For this review, take the finished solid that the model builds, in its own axes (mm). A direction names the side the tool comes from. Coordinates: 2 decimals unless noted, no trailing zeros. Order: outer loops, then holes, each group sorted by start corner. A loop starts at its lowest first (then second) coordinate and runs counter-clockwise, first axis right, second up. Notation, with made-up numbers: M -19,80.5 L -2,80.5 A23 cw -2,95.5 Z; hole C 2,74 d9. An arc over 180 degrees is marked long. Use CSV: the item, a comma, the result in double quotes.
```python
from build123d import *

# Parameters (mm, degrees)
F0_W      = 37.8
F0_H      = 23.2
F1_DEPTH  = 3
F3_DEPTH  = 4.5
F4_W      = 30
F4_H      = 13.9
F5_DEPTH  = 25.4
F4_W_2    = 34.5051246695
F4_H_2    = 1.524
F6_DEPTH  = 0.5
F7_R      = 0.25
F8_R      = 0.2
F9_R      = 0.2
F11_DEPTH = 5.5
F12_R     = 2.19964
F13_R     = 2.19964
F15_R     = 1.2
F14_R     = 1.2
F16_DEPTH = 25.4


with BuildPart() as f1:
    # F0 (on Top) → F1 (new body)
    with BuildSketch(Plane.XY):
        with Locations((18.9, 11.6)):
            Rectangle(F0_W, F0_H)
    extrude(amount=F1_DEPTH)

    # F2 (on face) → F3 (join)
    with BuildSketch(Plane.XY.offset(3)):
        Polygon((1.7535259355, 24.5575234294), (3.1678657052, 23.2), (3.544374615, 23.2), (2.1300348453, 24.5575234294), align=None)
        Polygon((3.544374615, 23.2), (3.1678657052, 23.2), (4.5401435345, 21.8828488141), (4.8160737062, 21.97938714), align=None)
        Polygon((2.5074673859, 0), (1.9109652349, 0), (1.0702608852, -0.7231329801), (1.3239181902, -1.0180314366), align=None)
        Polygon((4.5401435345, 1.7484091301), (4.5401435345, 2.2614912596), (1.9109652349, 0), (2.5074673859, 0), align=None)
        Polygon((33.6620093499, 2.2614912596), (35.6072341062, 0), (35.9434980693, 0), (33.998273313, 2.2614912596), align=None)
        Polygon((35.9434980693, 0), (35.6072341062, 0), (36.2292379141, -0.7231329801), (36.5655018772, -0.7231329801), align=None)
        Polygon((36.2128205597, 24.5575234294), (34.9098310654, 23.2), (35.2625123829, 23.2), (36.5655018772, 24.5575234294), align=None)
        Polygon((35.2625123829, 23.2), (34.9098310654, 23.2), (33.6403721345, 21.8774104865), (33.998273313, 21.8828488141), align=None)
    extrude(amount=F3_DEPTH)

    # F4 (on face) → F5 (cut)
    with BuildSketch(Plane(origin=(0, 0, 0), x_dir=(1, 0, 0), z_dir=(0, 0, -1))):
        with Locations((18.9, -11.6)):
            Rectangle(F4_W, F4_H)
    extrude(amount=-F5_DEPTH, mode=Mode.SUBTRACT)

    # F4 (on face) → F6 (cut)
    with BuildSketch(Plane(origin=(0, 0, 0), x_dir=(1, 0, 0), z_dir=(0, 0, -1))):
        with Locations((18.9, -11.6)):
            Rectangle(F4_W, F4_H)
        with Locations((18.9308619592, -1.8450859749)):
            Rectangle(F4_W_2, F4_H_2)
        with Locations((18.9308619592, -20.676838914)):
            Rectangle(F4_W_2, F4_H_2)
    extrude(amount=-F6_DEPTH, mode=Mode.SUBTRACT)

    # F7
    f7_edges = [f1.edges().sort_by_distance(p)[0] for p in [
        (18.930862, 2.607086, 0.5),
        (18.930862, 1.083086, 0.5),
        (18.930862, 19.914839, 0.5),
        (18.930862, 21.438839, 0.5),
        (1.6783, 19.914839, 0.25),
        (1.6783, 21.438839, 0.25),
        (1.6783, 2.607086, 0.25),
        (1.6783, 1.083086, 0.25),
        (1.6783, 1.845086, 0.5),
        (1.6783, 20.676839, 0.5),
        (36.183424, 19.914839, 0.25),
        (36.183424, 21.438839, 0.25),
        (36.183424, 20.676839, 0.5),
        (36.183424, 1.083086, 0.25),
        (36.183424, 2.607086, 0.25),
        (36.183424, 1.845086, 0.5),
    ]]
    fillet(f7_edges, radius=F7_R)

    # F8
    f8_edges = [f1.edges().sort_by_distance(p)[0] for p in [
        (18.930862, 1.083086, 0),
        (36.183424, 1.845086, 0),
        (36.110201, 1.156309, 0),
        (36.110201, 2.533863, 0),
        (1.6783, 1.845086, 0),
        (1.751523, 1.156309, 0),
        (1.751523, 2.533863, 0),
        (18.930862, 2.607086, 0),
    ]]
    fillet(f8_edges, radius=F8_R)

    # F9
    f9_edges = [f1.edges().sort_by_distance(p)[0] for p in [
        (18.930862, 19.914839, 0),
        (36.110201, 19.988062, 0),
        (36.183424, 20.676839, 0),
        (36.110201, 21.365616, 0),
        (18.930862, 21.438839, 0),
        (1.751523, 21.365616, 0),
        (1.6783, 20.676839, 0),
        (1.751523, 19.988062, 0),
    ]]
    fillet(f9_edges, radius=F9_R)

    # F10 (on face) → F11 (join)
    with BuildSketch(Plane(origin=(0, 23.2, 0), x_dir=(-1, 0, 0), z_dir=(0, 1, 0))):
        Polygon((-33.4, 2.5), (-33.4, 3), (-34.9098310654, 3), (-35.2625123829, 3), (-37.8, 3), (-37.8, 2.5), align=None)
        Polygon((0, 2.5), (0, 3), (-3.1678657052, 3), (-3.544374615, 3), (-4.4, 3), (-4.4, 2.5), align=None)
    extrude(amount=F11_DEPTH)

    # F12
    f12_edges = [f1.edges().sort_by_distance(p)[0] for p in [
        (0, 28.7, 2.75),
        (4.4, 28.7, 2.75),
    ]]
    fillet(f12_edges, radius=F12_R)

    # F13
    f13_edges = [f1.edges().sort_by_distance(p)[0] for p in [
        (33.4, 28.7, 2.75),
        (37.8, 28.7, 2.75),
    ]]
    fillet(f13_edges, radius=F13_R)

    # F15 (on face) + F14 (on face) → F16 (cut)
    with BuildSketch(Plane(origin=(0, 0, 2.5), x_dir=(1, 0, 0), z_dir=(0, 0, -1))):
        with Locations((2.2002029091, -26.3000000051)):
            Circle(F15_R)
    with BuildSketch(Plane(origin=(0, 0, 2.5), x_dir=(1, 0, 0), z_dir=(0, 0, -1))):
        with Locations((35.6002029091, -26.3000000051)):
            Circle(F14_R)
    extrude(amount=-F16_DEPTH, mode=Mode.SUBTRACT)


solid = f1.part
```
Item 1: Add section B-B on x = 13. State the section outline as (y, z) points, and give its area (3 significant figures).
Solutions:
outline,"M 0,0 L 0.88,0 A0.2 ccw 1.08,0.2 L 1.08,0.25 A0.25 cw 1.33,0.5 L 2.36,0.5 A0.25 cw 2.61,0.25 L 2.61,0.2 A0.2 ccw 2.81,0 L 4.65,0 L 4.65,3 L 0,3 Z; M 18.55,0 L 19.71,0 A0.2 ccw 19.91,0.2 L 19.91,0.25 A0.25 cw 20.16,0.5 L 21.19,0.5 A0.25 cw 21.44,0.25 L 21.44,0.2 A0.2 ccw 21.64,0 L 23.2,0 L 23.2,3 L 18.55,3 Z"
area,"26.4 mm^2"
Item 2: Add section C-C on z = 4. State the section outline as (x, y) points, and give its area (3 significant figures).
Solutions:
outline,"M 1.07,-0.72 L 1.32,-1.02 L 4.54,1.75 L 4.54,2.26 Z; M 1.75,24.56 L 4.54,21.88 L 4.82,21.98 L 2.13,24.56 Z; M 33.64,21.88 L 34,21.88 L 36.57,24.56 L 36.21,24.56 Z; M 33.66,2.26 L 36.23,-0.72 L 36.57,-0.72 L 34,2.26 Z"
area,"4.65 mm^2"
Item 3: For faces 1 (the face through (3.9, 12, 1)), 2 (the face through (2.2, 24.7, 2.5)), 3 (the face through (19, 2, 0.5)), 4 (the face through (3.77, 28.04, 2.75)), list the 3-axis set-ups (+Z, -Z, +X, -X, +Y, -Y) from which the entire face can be reached by the end or side of a thin tool; tool diameter is ignored.
Solutions:
face 1,"+Z, -Z"
face 2,"-Z, +X, -X, +Y"
face 3,"-Z"
face 4,"+Z, -Z, +Y"
Item 4: To check wall thickness, follow line 1 along Y through (x, z) = (31, 2); line 2 along Z through (x, y) = (12.5, 21.75); line 3 along X through (y, z) = (9.5, 0.5). State the ranges of each line that lie inside material, in increasing order. Write a range as [from, to].
Solutions:
line 1,"[0, 4.65], [18.55, 23.2]"
line 2,"[0, 3]"
line 3,"[0, 3.9], [33.9, 37.8]"
Item 5: Add section D-D on z = 1.5. State the section outline as (x, y) points, and give its area (3 significant figures).
Solutions:
outline,"M 0,0 L 37.8,0 L 37.8,23.2 L 0,23.2 Z; hole M 3.9,4.65 L 33.9,4.65 L 33.9,18.55 L 3.9,18.55 Z"
area,"460 mm^2"
Item 6: Draft analysis for pull direction X (two halves, no side actions). For faces 5 (the face through (0.63, 28.04, 2.75)), 6 (the face through (37.14, 28.07, 2.75)), 7 (the face through (19, 1, 3)), state which applies: released by +X, released by -X, zero draft, split by the parting line, or undercut.
Solutions:
face 5,"released by -X"
face 6,"released by +X"
face 7,"undercut"
Item 7: Add section A-A on y = 8.5. State the section outline as (x, z) points.
Solutions:
outline,"M 0,0 L 3.9,0 L 3.9,3 L 0,3 Z; M 33.9,0 L 37.8,0 L 37.8,3 L 33.9,3 Z"
Item 8: Clearance check with flat-ended pins moving along their axes: pin 1 Ø1.5 at (x, z) = (13.5, 2) entering from -Y; pin 2 Ø3 at (x, z) = (19, 3.5) entering from +Y; pin 3 Ø3.5 at (x, y) = (36.5, 25.5) entering from -Z; pin 4 Ø0.9 at (y, z) = (14, 1.5) entering from -X. State where each tip first meets the part, or that it passes through.
Solutions:
pin 1,"y = 0"
pin 2,"y = 23.2"
pin 3,"z = 2.5"
pin 4,"x = 0"
